Build history of the part. All positions in model axes, mm. Face numbers are marked on the shaded views. A direction names the side the tool comes from. Give positions to 0.01 mm unless a question says otherwise; leave off trailing zeros. Loops run counter-clockwise (first coordinate to the right, second up) from the corner with the lowest first, then second, coordinate; pieces in that order, holes last.
1) 3-axis set-ups, long thin cutter, end or side, ignore diameter. For the marked faces 1 and 2: which of +Z, -Z, +X, -X, +Y, -Y reach the whole face in a straight line?
2) Band-saw the part on D-D on x = -2. List the corners of the cut face in (y, z), then the cut area to 3 significant figures.
3) Two-plate mould, pull along Z, no slides. Class the marked faces 3, 4 and 5: +Z half, -Z half, draft (parallel to the pull), parting line (faces both ways), or undercut.
4) Wall check: line 1 (Z direction, x = -3.5, y = 7); line 2 (Y direction, x = -3, z = 0); line 3 (Z direction, x = 39, y = 7). Give the ranges that are in metal, low to high.
5) Band-saw the part on A-A on z = 0. List the corners of the cut face in (x, y), then the cut area to 3 significant figures.
6) Flat gauge pins, fed straight in: P1, Ø4.5, axis at y = 6.5, z = -0.5, coming from the +X side; P2, Ø6.5, axis at y = 8, z = 0, coming from the -X side. Where does each tip first touch, or does it go through?
7) Band-saw the part on C-C on x = 38. List the corners of the cut face in (y, z).
8) Band-saw the part on B-B on y = 7. List the corners of the cut face in (x, z).
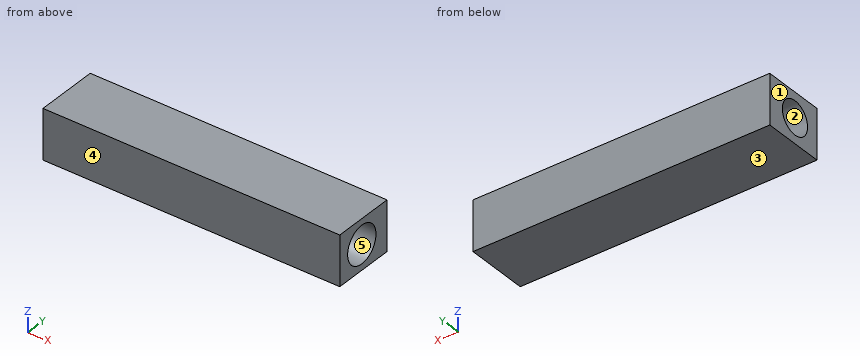
```python
from build123d import *

# Parameters (mm, degrees)
SKETCH_1_W          = 32.4
SKETCH_1_H          = 12
EXTRUDE_1_DEPTH     = 10
SKETCH_4_R          = 4
CUT_EXTRUDE_2_DEPTH = 8.5
SKETCH_7_R          = 3.4
CUT_EXTRUDE_3_DEPTH = 7.9
SKETCH_8_R          = 4.5
CUT_EXTRUDE_4_DEPTH = 16
SKETCH_9_W          = 32.4
SKETCH_9_H          = 2.645898034
EXTRUDE_2_DEPTH     = 5
EXTRUDE_3_DEPTH     = 5
EXTRUDE_4_DEPTH     = 5
SKETCH_12_W         = 12
SKETCH_12_H         = 5
EXTRUDE_5_DEPTH     = 32.4
SKETCH_13_R         = 4
CUT_EXTRUDE_5_DEPTH = 8.5
SKETCH_14_R         = 3.4
CUT_EXTRUDE_6_DEPTH = 7.9
SKETCH_15_R         = 4.5
CUT_EXTRUDE_8_DEPTH = 16
SKETCH_16_W         = 12
SKETCH_16_H         = 15
EXTRUDE_8_DEPTH     = 39
SKETCH_17_R         = 4.5
CUT_EXTRUDE_9_DEPTH = 39


with BuildPart() as part:
    # 草圖1 → 填料-伸長1 (new body)
    with BuildSketch(Plane(origin=(0, 0, 0), x_dir=(1, 0, 0), z_dir=(0, 1, 0))):
        Rectangle(SKETCH_1_W, SKETCH_1_H)
    extrude(amount=EXTRUDE_1_DEPTH)

    # 草圖4 → 除料-伸長2 (cut)
    with BuildSketch(Plane.ZY.offset(16.2)):
        with Locations((0, 7)):
            Circle(SKETCH_4_R)
    extrude(amount=-CUT_EXTRUDE_2_DEPTH, mode=Mode.SUBTRACT)

    # 草圖7 → 除料-伸長3 (cut)
    with BuildSketch(Plane.ZY.offset(7.7)):
        with Locations((0, 7)):
            Circle(SKETCH_7_R)
    extrude(amount=-CUT_EXTRUDE_3_DEPTH, mode=Mode.SUBTRACT)

    # 草圖8 → 除料-伸長4 (cut)
    with BuildSketch(Plane(origin=(16.2, 0, 0), x_dir=(0, 0, -1), z_dir=(1, 0, 0))):
        with Locations((0, 7)):
            Circle(SKETCH_8_R)
    extrude(amount=-CUT_EXTRUDE_4_DEPTH, mode=Mode.SUBTRACT)

    # 草圖9 → 填料-伸長2 (add)
    with BuildSketch(Plane(origin=(0, 10, 0), x_dir=(1, 0, 0), z_dir=(0, 1, 0))):
        with Locations((0, 4.677050983)):
            Rectangle(SKETCH_9_W, SKETCH_9_H)
    extrude(amount=EXTRUDE_2_DEPTH)

    # 草圖10 → 填料-伸長3 (add)
    with BuildSketch(Plane(origin=(0, 10, 0), x_dir=(1, 0, 0), z_dir=(0, 1, 0))):
        Polygon((-16.2, 3.372532617), (-16.2, 2.685476071), (-7.7, 2.645751311), (-7.7, 1.6), (0.2, 1.6), (0.2, 3.354101966), align=None)
    extrude(amount=EXTRUDE_3_DEPTH)

    # 草圖11 → 填料-伸長4 (add)
    with BuildSketch(Plane(origin=(0, 10, 0), x_dir=(1, 0, 0), z_dir=(0, 1, 0))):
        Polygon((-16.2, -2.660675208), (-16.2, -6), (16.2, -6), (16.2, -3.354101966), (0.2, -3.354101966), (0.2, -1.6), (-7.7, -1.6), (-7.7, -2.645751311), align=None)
    extrude(amount=EXTRUDE_4_DEPTH)

    # 草圖12 → 填料-伸長5 (add, through all)
    with BuildSketch(Plane.ZY.offset(16.2)):
        with Locations((0, 12.5)):
            Rectangle(SKETCH_12_W, SKETCH_12_H)
    extrude(amount=-EXTRUDE_5_DEPTH)

    # 草圖13 → 除料-伸長5 (cut)
    with BuildSketch(Plane.ZY.offset(16.2)):
        with Locations((0, 7)):
            Circle(SKETCH_13_R)
    extrude(amount=-CUT_EXTRUDE_5_DEPTH, mode=Mode.SUBTRACT)

    # 草圖14 → 除料-伸長6 (cut)
    with BuildSketch(Plane.ZY.offset(7.7)):
        with Locations((0, 7)):
            Circle(SKETCH_14_R)
    extrude(amount=-CUT_EXTRUDE_6_DEPTH, mode=Mode.SUBTRACT)

    # 草圖15 → 除料-伸長8 (cut)
    with BuildSketch(Plane(origin=(16.2, 0, 0), x_dir=(0, 0, -1), z_dir=(1, 0, 0))):
        with Locations((0, 7)):
            Circle(SKETCH_15_R)
    extrude(amount=-CUT_EXTRUDE_8_DEPTH, mode=Mode.SUBTRACT)

    # 草圖16 → 填料-伸長8 (add)
    with BuildSketch(Plane(origin=(16.2, 0, 0), x_dir=(0, 0, -1), z_dir=(1, 0, 0))):
        with Locations((0, 7.5)):
            Rectangle(SKETCH_16_W, SKETCH_16_H)
    extrude(amount=EXTRUDE_8_DEPTH)

    # 草圖17 → 除料-伸長9 (cut)
    with BuildSketch(Plane(origin=(55.2, 0, 0), x_dir=(0, 0, -1), z_dir=(1, 0, 0))):
        with Locations((0, 7)):
            Circle(SKETCH_17_R)
    extrude(amount=-CUT_EXTRUDE_9_DEPTH, mode=Mode.SUBTRACT)


solid = part.part
```
Findings below:
1. face 1: +Z, -Z, -X, +Y, -Y
1. face 2: -X
2. outline: (0, -6) - (15, -6) - (15, 6) - (0, 6) - close; hole circle Ø6.8 at (7, 0)
2. area: 144 mm2
3. face 3: -Z half
3. face 4: draft
3. face 5: undercut
4. line 1: z = -6 to -3.4, 3.4 to 6
4. line 2: y = 0 to 3.6, 10.4 to 15
4. line 3: z = -6 to -4.5, 4.5 to 6
5. outline: (-16.2, 0) - (55.2, 0) - (55.2, 2.5) - (0.2, 2.5) - (0.2, 3.6) - (-7.7, 3.6) - (-7.7, 3) - (-16.2, 3) - close; (-16.2, 11) - (-7.7, 11) - (-7.7, 10.4) - (0.2, 10.4) - (0.2, 11.5) - (55.2, 11.5) - (55.2, 15) - (-16.2, 15) - close
5. area: 454 mm2
6. P1: passes through
6. P2: stops at x = -16.2
7. outline: (0, -6) - (15, -6) - (15, 6) - (0, 6) - close; hole circle Ø9 at (7, 0)
8. outline: (-16.2, -6) - (55.2, -6) - (55.2, -4.5) - (0.2, -4.5) - (0.2, -3.4) - (-7.7, -3.4) - (-7.7, -4) - (-16.2, -4) - close; (-16.2, 4) - (-7.7, 4) - (-7.7, 3.4) - (0.2, 3.4) - (0.2, 4.5) - (55.2, 4.5) - (55.2, 6) - (-16.2, 6) - close
